Can you work these out from the model? Positions are in its coordinate system, mm. Coordinates: 2 decimals unless noted, no trailing zeros. Order: outer loops, then holes, each group sorted by start corner. A loop starts at its lowest first (then second) coordinate and runs counter-clockwise, first axis right, second up.
```python
from build123d import *

# Parameters (mm, degrees)
SKETCH1_W           = 324.5
SKETCH1_H           = 394
BOSS_EXTRUDE1_DEPTH = 5
SKETCH2_R           = 2.5
CUT_EXTRUDE1_DEPTH  = 256.262732298
SKETCH4_R           = 5
CUT_EXTRUDE3_DEPTH  = 5
SKETCH5_R           = 2.5
CUT_EXTRUDE4_DEPTH  = 5
SKETCH7_R           = 15
SKETCH7_R_2         = 3.75
CUT_EXTRUDE6_DEPTH  = 256.262732298


with BuildPart() as part:
    # Sketch1 → Boss-Extrude1 (new body)
    with BuildSketch(Plane.XY):
        Rectangle(SKETCH1_W, SKETCH1_H)
    extrude(amount=BOSS_EXTRUDE1_DEPTH)

    # Sketch2 → Cut-Extrude1 (cut, through all)
    with BuildSketch(Plane.XY.offset(5)):
        with Locations((152.25, 187)):
            Circle(SKETCH2_R)
        with Locations((-152.25, 187)):
            Circle(SKETCH2_R)
        with Locations((-152.25, -187)):
            Circle(SKETCH2_R)
        with Locations((152.25, -187)):
            Circle(SKETCH2_R)
    extrude(amount=-CUT_EXTRUDE1_DEPTH, mode=Mode.SUBTRACT)

    # Sketch4 → Cut-Extrude3 (cut)
    with BuildSketch(Plane(origin=(0, 0, 0), x_dir=(-1, 0, 0), z_dir=(0, 0, -1))):
        with Locations((80.422215232, 65)):
            Circle(SKETCH4_R)
        with Locations((136.713866478, 32.5)):
            Circle(SKETCH4_R)
        with Locations((136.713866478, -32.5)):
            Circle(SKETCH4_R)
        with Locations((80.422215232, -65)):
            Circle(SKETCH4_R)
        with Locations((24.130563986, -32.5)):
            Circle(SKETCH4_R)
        with Locations((24.130563986, 32.5)):
            Circle(SKETCH4_R)
    extrude(amount=-CUT_EXTRUDE3_DEPTH, mode=Mode.SUBTRACT)

    # Sketch5 → Cut-Extrude4 (cut)
    with BuildSketch(Plane.XY.offset(5)):
        with Locations((38.192392445, 12)):
            Circle(SKETCH5_R)
        with Locations((50.192392445, 0)):
            Circle(SKETCH5_R)
        with Locations((38.192392445, -12)):
            Circle(SKETCH5_R)
        with Locations((26.192392445, 0)):
            Circle(SKETCH5_R)
    extrude(amount=-CUT_EXTRUDE4_DEPTH, mode=Mode.SUBTRACT)

    # Sketch7 → Cut-Extrude6 (cut, through all)
    with BuildSketch(Plane(origin=(0, 0, 0), x_dir=(-1, 0, 0), z_dir=(0, 0, -1))):
        with Locations((-109.31, 167)):
            Circle(SKETCH7_R)
        with Locations((-109.31, -167)):
            Circle(SKETCH7_R)
        with Locations((-109.31, 189.5)):
            Circle(SKETCH7_R_2)
        with Locations((-109.31, -144.5)):
            Circle(SKETCH7_R_2)
        with Locations((-86.81, -167)):
            Circle(SKETCH7_R_2)
        with Locations((-109.31, -189.5)):
            Circle(SKETCH7_R_2)
        with Locations((-131.81, -167)):
            Circle(SKETCH7_R_2)
        with Locations((-86.81, 167)):
            Circle(SKETCH7_R_2)
        with Locations((-109.31, 144.5)):
            Circle(SKETCH7_R_2)
        with Locations((-131.81, 167)):
            Circle(SKETCH7_R_2)
    extrude(amount=-CUT_EXTRUDE6_DEPTH, mode=Mode.SUBTRACT)


solid = part.part
```
1. Imagine slicing it at B-B on y = 65. Please give me the cut outline in (x, z), then the cut area to 3 significant figures.
Completed:
outline: (-162.25, 0) - (-85.42, 0) - (-85.42, 5) - (-162.25, 5) - close; (-75.42, 0) - (162.25, 0) - (162.25, 5) - (-75.42, 5) - close
area: 1,570 mm2
2. I'm going to push flat-ended pins straight in: pin 1 (8 mm diameter, centred on x = 38.19, y = -12, fed in from +Z); pin 2 (7 mm diameter, centred on x = 109.31, y = 189.5, fed in from +Z). Where does each tip first touch, or does it pass through?
Completed:
pin 1: stops at z = 5
pin 2: passes through
3. Imagine slicing it at A-A on z = 1.2. Give the number of separate pieces and of enclosed holes in the cut face, then the cut area to 3 significant figures.
Completed:
separate pieces: 1
enclosed holes: 24
area: 125,000 mm2
4. Please list where these lines run through material, in increasing order: probe 1 along Y at (x, z) = (152.25, 3); probe 2 along Y at (x, z) = (-28.5, 3.95); probe 3 along X at (y, z) = (187, 1.85).
Completed:
probe 1: y = -197 to -189.5, -184.5 to 184.5, 189.5 to 197
probe 2: y = -197 to -34.93, -30.07 to 30.07, 34.93 to 197
probe 3: x = -162.25 to -154.75, -149.75 to 106.51, 112.11 to 149.75, 154.75 to 162.25
5. Thinking about a two-plate mould opening in X: for faces 1 (the flat face through (-2, 3, 0)), 2 (the cylindrical face through (-20.16, -35.54, 2.46)), which applies, pulls with the +X half, pulls with the -X half, needs draft (parallel to the pull), parting line crosses it, or undercut?
Completed:
face 1: needs draft
face 2: undercut
